from build123d import *

# Parameters (mm, degrees)
SKETCH3_R                    = 9.825
LENS_TOP_CUT_EXTRUDE2_DEPTH  = 0.91
SKETCH2_W                    = 1
SKETCH2_H                    = 0.861432774
TOP_CUT_EXTRUDE3_DEPTH       = 1.4
BOTTOM_CUT_EXTRUDE4_DEPTH    = 0.8
SIDE_CUT_EXTRUDE5_DEPTH      = 8
SKETCH6_R                    = 2.6
LENS_HOLE_CUT_EXTRUDE7_DEPTH = 5


with BuildPart() as part:
    # Sketch1 → Lens Holder (revolve)
    with BuildSketch(Plane.XY, mode=Mode.PRIVATE) as lens_holder_sk:
        with BuildLine():
            Line((0, 0), (4.975, 0))
            Line((4.975, 0), (4.975, 0.65))
            ThreePointArc((4.975, 0.65), (8.271800133, 4.752191856), (10.5, 9.52))
            Line((10.5, 9.52), (10.5, 12.72))
            Line((10.5, 12.72), (0, 12.72))
            Line((0, 12.72), (0, 0))
        make_face()
    revolve(lens_holder_sk.sketch.rotate(Axis((0, 0, 0), (0, 1, 0)), 90), axis=Axis((0, 0, 0), (0, 1, 0)))

    # Sketch3 → Lens Top Cut-Extrude2 (cut)
    with BuildSketch(Plane(origin=(0, 12.72, 0), x_dir=(1, 0, 0), z_dir=(0, 1, 0))):
        with Locations(Location((0, 0, 0), (0, 0, 270))):
            Circle(SKETCH3_R)
    extrude(amount=-LENS_TOP_CUT_EXTRUDE2_DEPTH, mode=Mode.SUBTRACT)

    # Sketch2 → Top Cut-Extrude3 (cut)
    with BuildSketch(Plane(origin=(0, 12.72, 0), x_dir=(1, 0, 0), z_dir=(0, 1, 0))):
        Polygon((8.40360039, -6.29519662), (7.90360039, -7.161222024), (7.157577724, -6.730505637), (7.657577724, -5.864480233), align=None)
        with Locations((1.75, 9.994613344)):
            Rectangle(SKETCH2_W, SKETCH2_H)
        with Locations((-1.75, 9.994613344)):
            Rectangle(SKETCH2_W, SKETCH2_H)
        Polygon((10.15360039, -3.264107707), (9.65360039, -4.130133111), (8.907577724, -3.699416724), (9.407577724, -2.83339132), align=None)
        Polygon((-9.65360039, -4.130133111), (-10.15360039, -3.264107707), (-9.407577724, -2.83339132), (-8.907577724, -3.699416724), align=None)
        Polygon((-7.90360039, -7.161222024), (-8.40360039, -6.29519662), (-7.657577724, -5.864480233), (-7.157577724, -6.730505637), align=None)
    extrude(amount=-TOP_CUT_EXTRUDE3_DEPTH, mode=Mode.SUBTRACT)

    # Sketch4 → Bottom Cut-Extrude4 (cut)
    with BuildSketch(Plane.XZ):
        Polygon((2.49, 1.8), (1.99, 1.3), (2.49, 0.8), (2.49, -0.8), (1.99, -1.3), (2.49, -1.8), (2.49, -2.49), (1.8, -2.49), (1.3, -1.99), (0.8, -2.49), (-0.8, -2.49), (-1.3, -1.99), (-1.8, -2.49), (-2.49, -2.49), (-2.49, -1.8), (-1.99, -1.3), (-2.49, -0.8), (-2.49, 0.8), (-1.99, 1.3), (-2.49, 1.8), (-2.49, 2.49), (-1.8, 2.49), (-1.3, 1.99), (-0.8, 2.49), (0.8, 2.49), (1.3, 1.99), (1.8, 2.49), (2.49, 2.49), align=None)
    extrude(amount=-BOTTOM_CUT_EXTRUDE4_DEPTH, mode=Mode.SUBTRACT)

    # Sketch5 → Side Cut-Extrude5 (cut)
    with BuildSketch(Plane(origin=(0, 9.52, 0), x_dir=(1, 0, 0), z_dir=(0, 1, 0))):
        with BuildLine():
            Line((-1.3, 10.01598722), (-1.3, 8.1))
            Line((-1.3, 8.1), (1.3, 8.1))
            Line((1.3, 8.1), (1.3, 10.01598722))
            ThreePointArc((1.3, 10.01598722), (0, 10.1), (-1.3, 10.01598722))
        make_face()
        with BuildLine():
            Line((8.024099377, -6.133826635), (6.364805771, -5.175833025))
            Line((6.364805771, -5.175833025), (7.664805771, -2.924166975))
            Line((7.664805771, -2.924166975), (9.324099377, -3.882160585))
            ThreePointArc((9.324099377, -3.882160585), (8.746856578, -5.05), (8.024099377, -6.133826635))
        make_face()
        with BuildLine():
            Line((-9.324099377, -3.882160585), (-7.664805771, -2.924166975))
            Line((-7.664805771, -2.924166975), (-6.364805771, -5.175833025))
            Line((-6.364805771, -5.175833025), (-8.024099377, -6.133826635))
            ThreePointArc((-8.024099377, -6.133826635), (-8.746856578, -5.05), (-9.324099377, -3.882160585))
        make_face()
    extrude(amount=-SIDE_CUT_EXTRUDE5_DEPTH, mode=Mode.SUBTRACT)

    # Sketch6 → Lens Hole Cut-Extrude7 (cut)
    with BuildSketch(Plane.XZ.offset(-0.8)):
        with Locations(Location((0, 0, 0), (0, 0, 270))):
            Circle(SKETCH6_R)
    extrude(amount=-LENS_HOLE_CUT_EXTRUDE7_DEPTH, mode=Mode.SUBTRACT)


solid = part.part
Can you work these out from the model? Positions are in its coordinate system, mm. A direction names the side the tool comes from. Coordinates: 2 decimals unless noted, no trailing zeros. Put each result on its own line as item: value. Start each with the question number.
Item 1: Which directions (+Z, -Z, +X, -X, +Y, -Y) give clear straight access to the entire face, cutting with the end or side of a thin tool? Please do faces 4 (the face through (-0.112, 12.271, 9.824)), 5 (the face through (2, 11.32, -10)), 6 (the face through (2, 0.8, 2)).
Item 2: For pin 1 (0.5 mm diameter, centred on x = 2, z = -2, fed in from -Y); pin 2 (2 mm diameter, centred on x = 2.5, y = 7, fed in from -Z); pin 3 (0.7 mm diameter, centred on y = 12, z = -10, fed in from +X), each with a flat end and sliding along its axis, tell me the tip position at first contact or that it passes through.
Item 3: Suppose I cut it at A-A (y = 9). State how many separate pieces and enclosed holes the cut face has, and give its area (3 significant figures).
Item 4: If we mould it in two halves opening along Z, with no side actions, what happens to faces 1 (the face through (-2, 11.32, -10)), 2 (the face through (3.027, 0.33, 3.948)), 3 (the face through (0, 9.52, -9))? For each: +Z half, -Z half, draft (parallel to the pull), parting line (faces both ways), or undercut.
Item 5: If I drill on line 1 along Y through (x, z) = (1, -3.25); line 2 along X through (y, z) = (9, 2.5); line 3 along X through (y, z) = (3.7, 0), over which ranges is the centre line in solid material (lowest first)?
Here are the results:
1. face 4: +Y
1. face 5: -Z, +Y
1. face 6: -Y
2. pin 1: y = 0.8
2. pin 2: z = -9.68
2. pin 3: x = 4.14
3. separate pieces: 1
3. enclosed holes: 3
3. area: 319 mm²
4. face 1: draft
4. face 2: parting line
4. face 3: undercut
5. line 1: 0 to 11.81
5. line 2: -10.01 to 10.01
5. line 3: -7.57 to -2.6, 2.6 to 7.57
